```python
from build123d import *

# Parameters (mm, degrees)
BOSS_EXTRUDE1_DEPTH = 5
SKETCH2_W           = 6.5
SKETCH2_H           = 17
CUT_EXTRUDE1_DEPTH  = 20
CUT_EXTRUDE2_DEPTH  = 2.5
SKETCH4_R           = 1.75
CUT_EXTRUDE3_DEPTH  = 10
BOSS_EXTRUDE2_DEPTH = 1.5


with BuildPart() as part:
    # Sketch1 → Boss-Extrude1 (new, symmetric)
    with BuildSketch(Plane(origin=(0, 0, 0), x_dir=(0, 0, -1), z_dir=(1, 0, 0))):
        with BuildLine():
            Line((-6, 0), (6, 0))
            Line((6, 0), (6, 12))
            Line((6, 12), (0.901387819, 13.5))
            ThreePointArc((0.901387819, 13.5), (-1.75, 15), (0.901387819, 16.5))
            Line((0.901387819, 16.5), (6, 18))
            Line((6, 18), (6, 26))
            Line((6, 26), (-6, 26))
            Line((-6, 26), (-6, 0))
        make_face()
    extrude(amount=BOSS_EXTRUDE1_DEPTH, both=True)

    # Sketch2 → Cut-Extrude1 (cut)
    with BuildSketch(Plane.XY.offset(6)):
        with Locations((0, 15)):
            Rectangle(SKETCH2_W, SKETCH2_H)
    extrude(amount=-CUT_EXTRUDE1_DEPTH, mode=Mode.SUBTRACT)

    # Sketch3 → Cut-Extrude2 (cut)
    with BuildSketch(Plane.XY):
        Polygon((-2.75, 0), (2.75, 0), (2.75, 5.184123402), (0, 6.771836642), (-2.75, 5.184123402), align=None)
    extrude(amount=-CUT_EXTRUDE2_DEPTH, mode=Mode.SUBTRACT)

    # Sketch4 → Cut-Extrude3 (cut, symmetric)
    with BuildSketch(Plane.XY):
        with Locations(Location((0, 3.25, 0), (0, 0, 180))):
            Circle(SKETCH4_R)
    extrude(amount=CUT_EXTRUDE3_DEPTH, both=True, mode=Mode.SUBTRACT)

    # Sketch5 → Boss-Extrude2 (add, symmetric)
    with BuildSketch(Plane(origin=(0, 0, 0), x_dir=(0, 0, -1), z_dir=(1, 0, 0))):
        with BuildLine():
            Line((6, 5), (6, 6.5))
            ThreePointArc((6, 6.5), (9.25, 3.25), (6, 0))
            Line((6, 0), (6, 1.5))
            ThreePointArc((6, 1.5), (7.75, 3.25), (6, 5))
        make_face()
        with BuildLine():
            Line((-4.4, 0), (-6, 0))
            ThreePointArc((-6, 0), (-3, -3), (0, 0))
            Line((0, 0), (-1.6, 0))
            ThreePointArc((-1.6, 0), (-3, -1.4), (-4.4, 0))
        make_face()
    extrude(amount=BOSS_EXTRUDE2_DEPTH, both=True)


solid = part.part
```
Build history of the part. All positions in model axes, mm. A direction names the side the tool comes from. Give positions to 0.01 mm unless a question says otherwise; leave off trailing zeros. Loops run counter-clockwise (first coordinate to the right, second up) from the corner with the lowest first, then second, coordinate; pieces in that order, holes last. Notation, with made-up numbers: (-36, 46) -> (4, 46) arc R28 cw to (4, 71) -> close; hole circle Ø10 at (-19.75, -22.75). An arc over 180 degrees is marked (long way). One line per question, with ' | ' between items.
Q1. Cut at B-B, the plane y = 3.25. Write the cut outline in (x, z), plus the area to 3 significant figures.
Filled sheet:
outline: (-5, -6) -> (-1.75, -6) -> (-1.75, -2.5) -> (-2.75, -2.5) -> (-2.75, 0) -> (-1.75, 0) -> (-1.75, 6) -> (-5, 6) -> close; (-1.5, -9.25) -> (1.5, -9.25) -> (1.5, -7.75) -> (-1.5, -7.75) -> close; (1.75, -6) -> (5, -6) -> (5, 6) -> (1.75, 6) -> (1.75, 0) -> (2.75, 0) -> (2.75, -2.5) -> (1.75, -2.5) -> close | area: 77.5 mm²
Q2. Cut at A-A, the plane y = 15. Write the cut outline in (x, z), plus the area to 3 significant figures.
Filled sheet:
outline: (-5, 1.75) -> (-3.25, 1.75) -> (-3.25, 6) -> (-5, 6) -> close; (3.25, 1.75) -> (5, 1.75) -> (5, 6) -> (3.25, 6) -> close | area: 14.9 mm²
Q3. Drill centre lines: line 1 along Y through (x, z) = (2.5, 3.75); line 2 along Y through (x, z) = (0, -3.7); line 3 along X through (y, z) = (12, -2). Where is each one in solid material? Low to high. Write a range as [from, to].
Filled sheet:
line 1: y = [0, 6.5], [23.5, 26] | line 2: y = [0, 1.5], [5, 6.5], [23.5, 26] | line 3: x = [-5, -3.25], [3.25, 5]
Q4. Cut at D-D, the plane z = -8.25. Write the cut outline in (x, y).
Filled sheet:
outline: (-1.5, 0.9) -> (1.5, 0.9) -> (1.5, 5.6) -> (-1.5, 5.6) -> close
Q5. Drop flat-ended pins along their axis: pin 1 (2.5 mm diameter, centred on x = -3, y = 6.5, fed in from -Z); pin 2 (2.5 mm diameter, centred on y = 4.5, z = -8, fed in from +X); pin 3 (2.5 mm diameter, centred on x = 2.5, y = 5.5, fed in from -Z). Give the stop position or say it passes through.
Filled sheet:
pin 1: stops at z = -6 | pin 2: stops at x = 1.5 | pin 3: stops at z = -8.88
Q6. Cut at C-C, the plane y = 10.75. Write the cut outline in (x, z).
Filled sheet:
outline: (-5, -6) -> (-3.25, -6) -> (-3.25, 6) -> (-5, 6) -> close; (3.25, -6) -> (5, -6) -> (5, 6) -> (3.25, 6) -> close
Q7. Pull direction X, two halves, no side cores. Call faces 1 (the flat face through (1.5, -2, 3)), 2 (the flat face through (-4.11, 12.74, -3.49)), 3 (the flat face through (-2.75, 3, -1)): pulls with the +X half, pulls with the -X half, needs draft (parallel to the pull), parting line crosses it, or undercut.
Filled sheet:
face 1: pulls with the +X half | face 2: needs draft | face 3: undercut
Q8. Tool access for faces 4 (the flat face through (-1.5, 3, -8)), 5 (the flat face through (0, 1, 0)), 6 (the cylindrical face through (0, 5, 3)), 7 (the flat face through (1.5, 3, -8)): list every direction of +Z, -Z, +X, -X, +Y, -Y with a clear straight run to the whole face (end or side of a thin tool).
Filled sheet:
face 4: -Z, -X, +Y, -Y | face 5: -Y | face 6: +Z | face 7: -Z, +X, +Y, -Y
